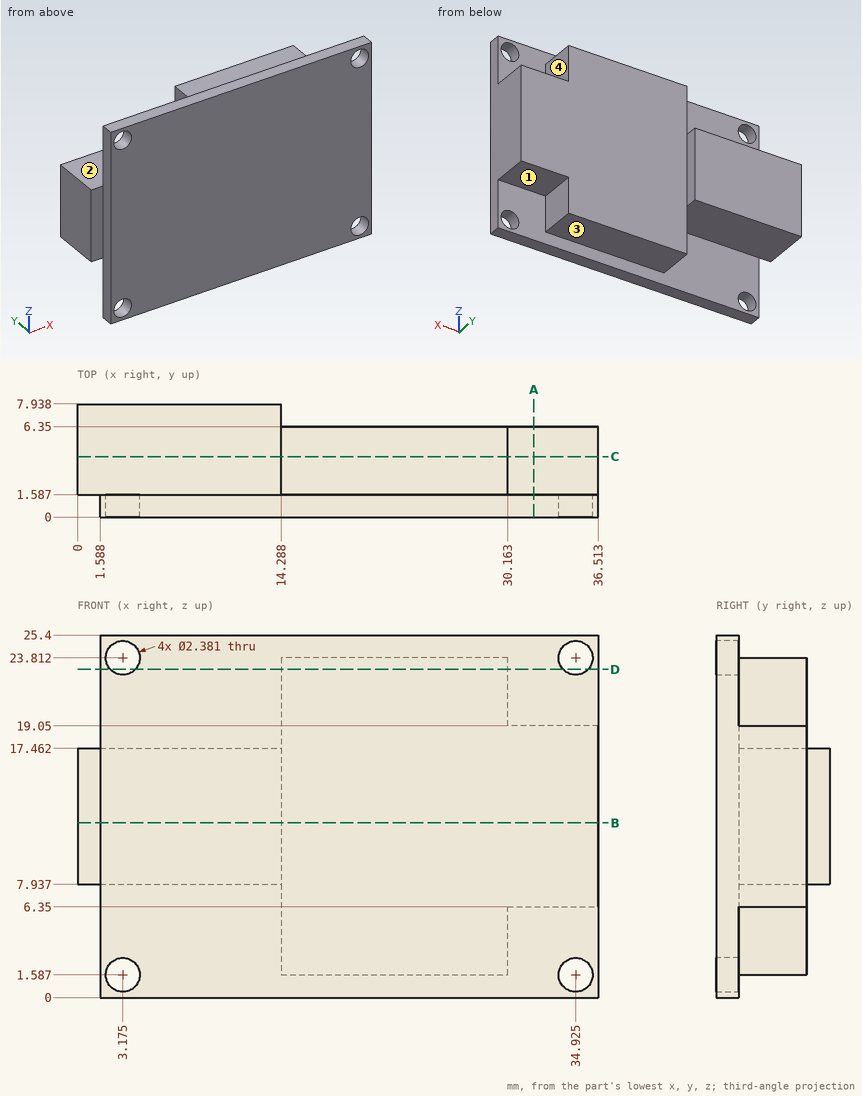
Drawing for the job (mm, zero at the part's lowest x, y, z). A direction names the side the tool comes from. Round coordinates to 2 decimals unless told otherwise and drop trailing zeros. Write each loop counter-clockwise with the first axis right and the second up, starting at its lowest first coordinate (ties: lowest second). Pieces come first, ordered by that corner, then holes. Notation, with made-up numbers: M 83.5,60 L 130.5,60 A27 ccw 130.5,76 Z; hole C 5,-22 d8. An arc over 180 degrees is marked long. Answer as a JSON object with one key per item and string values. Group by question number.
(1) Drill centre lines: L1, parallel to Z at x = 23, y = 3; L2, parallel to Z at x = 2, y = 2.5; L3, parallel to Z at x = 3.5, y = 0.75. Where is each one in solid material? Low to high.
(2) Cut at D-D (z = 23). Give the number of separate pieces and of enclosed holes in the cut face.
(3) Cut at A-A (x = 32). Give the cut face in (y, z), and give its area (3 significant figures).
(4) Cut at B-B (z = 12.25). Give the cut face in (x, y).
(5) Cut at C-C (y = 4.25). Give the cut face in (x, z).
(6) Flat gauge pins, fed straight in: pin 1 (2 mm diameter, centred on x = 34.92, z = 1.59, fed in from +Y); pin 2 (2.5 mm diameter, centred on y = 3, z = 4.5, fed in from -X); pin 3 (3 mm diameter, centred on x = 21.5, y = 6.5, fed in from -Z); pin 4 (3 mm diameter, centred on x = 10, y = 4, fed in from -Z). Where does each tip first touch, or does it go through?
(7) Which spindle directions (+Z, -Z, +X, -X, +Y, -Y) get a long thin tool onto all of the face, cutting with end or side? Do the marked faces 1, 2, 3 and 4. Say none if no direction does.
Responses:
{
 "1": {"L1": "z = 1.59 to 23.81", "L2": "z = 7.94 to 17.46", "L3": "z = 0 to 0.44, 2.73 to 22.67, 24.96 to 25.4"},
 "2": {"separate pieces": "3", "enclosed holes": "0"},
 "3": {"outline": "M 0,0 L 1.59,0 L 1.59,6.35 L 6.35,6.35 L 6.35,19.05 L 1.59,19.05 L 1.59,25.4 L 0,25.4 Z", "area": "101 mm2"},
 "4": {"outline": "M 0,1.59 L 1.59,1.59 L 1.59,0 L 36.51,0 L 36.51,6.35 L 14.29,6.35 L 14.29,7.94 L 0,7.94 Z"},
 "5": {"outline": "M 0,7.94 L 14.29,7.94 L 14.29,1.59 L 30.16,1.59 L 30.16,6.35 L 36.51,6.35 L 36.51,19.05 L 30.16,19.05 L 30.16,23.81 L 14.29,23.81 L 14.29,17.46 L 0,17.46 Z"},
 "6": {"pin 1": "passes through", "pin 2": "stops at x = 14.29", "pin 3": "stops at z = 1.59", "pin 4": "stops at z = 7.94"},
 "7": {"face 1": "-Z, +X, +Y", "face 2": "+Z, -X, +Y", "face 3": "-Z, +X, -X, +Y", "face 4": "+Z, +X, +Y"}
}
